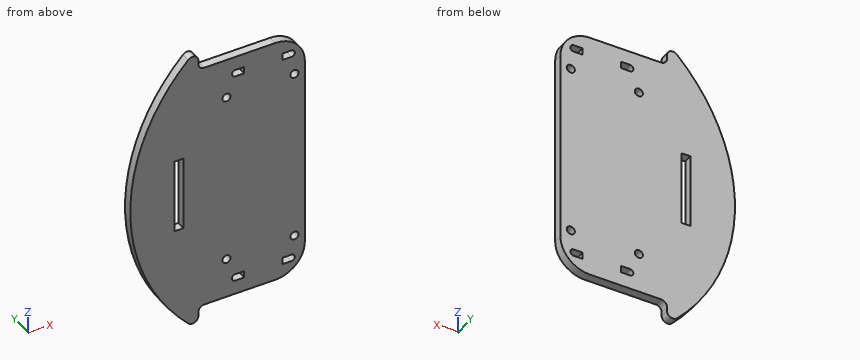
Autodesk Inventor part; units mm, degrees
ref_plane "YZ Plane" through (0, 0, 0) normal (1, 0, 0) x (0, 1, 0)
ref_plane "XZ Plane" through (0, 0, 0) normal (0, 1, 0) x (-1, 0, 0)
ref_plane "XY Plane" through (0, 0, 0) normal (0, 0, 1) x (1, 0, 0)
sketch "Boceto1" plane through (0, 0, 0) normal (0, 1, 0) x (-1, 0, 0)
  line L0 (3, 0) -> (33, 0)
  line L1 (36, -3) -> (36, -62)
  line L2 (33, -65) -> (3, -65)
  line L3 (0, -62) -> (0, -3)
  circle A0 centre (3.5, -61.5) radius 1.375
  arc A1 (36, -3) -> (33, 0) centre (33, -3) ccw
  arc A2 (3, 0) -> (0, -3) centre (3, -3) ccw
  arc A3 (0, -62) -> (3, -65) centre (3, -62) ccw
  arc A4 (33, -65) -> (36, -62) centre (33, -62) ccw
  circle A5 centre (26.5, -61.5) radius 1.375
  circle A6 centre (3.5, -3.5) radius 1.375
  circle A7 centre (26.5, -3.5) radius 1.375
  line L4 (36, 0) -> (0, 0)
  line L5 (0, 0) -> (0, 10)
  line L6 (0, 10) -> (36, 10)
  line L7 (36, 10) -> (36, 0)
  line L8 (36, -65) -> (0, -65)
  line L9 (0, -65) -> (0, -75)
  line L10 (0, -75) -> (36, -75)
  line L11 (36, -75) -> (36, -65)
  line L12 (7.5, 0) -> (20.5, 0)
  line L13 (20.5, 0) -> (20.5, 10)
  line L14 (20.5, 10) -> (7.5, 10)
  line L15 (7.5, 10) -> (7.5, 0)
  line L16 (7.5, 0) -> (20.5, 10) construction
  line L17 (20.5, 0) -> (7.5, 10) construction
  line L18 (7.5, -75) -> (20.5, -75)
  line L19 (20.5, -75) -> (20.5, -65)
  line L20 (20.5, -65) -> (7.5, -65)
  line L21 (7.5, -65) -> (7.5, -75)
  line L22 (7.5, -75) -> (20.5, -65) construction
  line L23 (20.5, -75) -> (7.5, -65) construction
  line L24 (36, -32.5) -> (0, -32.5)
  line L25 (36, 0) -> (36, -3)
  line L26 (0, 0) -> (0, -3)
  line L27 (0, -62) -> (0, -65)
  line L28 (36, -62) -> (36, -65)
  line L29 (36, -22.5) -> (49, -22.5)
  line L30 (49, -22.5) -> (49, -42.5)
  line L31 (49, -42.5) -> (36, -42.5)
  line L32 (36, -42.5) -> (36, -22.5)
  arc A8 (49, -42.5) -> (49, -22.5) centre (49, -32.5) ccw
  line L33 (20.5, 5.3) -> (23.5, 5.3)
  line L34 (23.5, 5.3) -> (23.5, 3)
  line L35 (23.5, 3) -> (20.5, 3)
  line L36 (20.5, 3) -> (20.5, 5.3)
  arc A9 (23.5, 3) -> (23.5, 5.3) centre (23.5, 4.15) ccw
  line L37 (14, 0) -> (14, -65)
  line L38 (7.5, 5.3) -> (4.5, 5.3)
  line L39 (4.5, 5.3) -> (4.5, 3)
  line L40 (4.5, 3) -> (7.5, 3)
  line L41 (7.5, 3) -> (7.5, 5.3)
  arc A10 (4.5, 5.3) -> (4.5, 3) centre (4.5, 4.15) ccw
  line L42 (20.5, -70.3) -> (23.5, -70.3)
  line L43 (23.5, -70.3) -> (23.5, -68)
  line L44 (23.5, -68) -> (20.5, -68)
  line L45 (20.5, -68) -> (20.5, -70.3)
  arc A11 (23.5, -70.3) -> (23.5, -68) centre (23.5, -69.15) ccw
  line L46 (4.5, -68) -> (7.5, -68)
  arc A12 (4.5, -68) -> (4.5, -70.3) centre (4.5, -69.15) ccw
  line L47 (7.5, -70.3) -> (4.5, -70.3)
  line L48 (4.5, -70.3) -> (4.5, -68)
  line L49 (7.5, -68) -> (7.5, -70.3)
  line L50 (36, 0) -> (49, 0)
  line L51 (49, 0) -> (49, -65)
  line L52 (49, -65) -> (36, -65)
  line L53 (36, -65) -> (36, 0)
  line L54 (44, -20) -> (41, -20)
  line L55 (41, -20) -> (41, -45)
  line L56 (41, -45) -> (44, -45)
  line L57 (44, -45) -> (44, -20)
  line L58 (36, 10) -> (36, 18)
  line L59 (36, -75) -> (36, -83)
  arc A13 (36, -83) -> (36, 18) centre (-7.9402, -32.5) ccw
  line L60 (0, -75) -> (-7, -75)
  line L61 (-7, -75) -> (-7, 10)
  line L62 (-7, 10) -> (0, 10)
  line L63 (0, 10) -> (0, -75)
  point P0 (14, 5)
  point P1 (14, -70)
  point P2 (36, -42.5)
  point P3 (7.5, -70.3)
  point P4 (20.5, -70.3)
  point P5 (7.5, 5.3)
  point P6 (20.5, 3)
  point P7 (44, -32.5)
  point P8 (36, -65)
  point P9 (44, -42.5)
  point P10 (41, -42.5)
  point P11 (41, -22.5)
  point P12 (44, -22.5)
  point P13 (49, -22.5)
  point P14 (59, -32.5)
  dimension "d0" = 36
  dimension "d1" = 65
  dimension "d2" = 2.75
  dimension "d3" = 3
  dimension "d4" = 3
  dimension "d5" = 3
  dimension "d6" = 3
  dimension "d7" = 3.5
  dimension "d8" = 3.5
  dimension "d11" = 23
  dimension "d14" = 58
  dimension "d17" = 10
  dimension "d18" = 10
  dimension "d19" = 13
  dimension "d20" = 10
  dimension "d21" = 13
  dimension "d22" = 10
  dimension "d26" = 7.5
  dimension "d30" = 20
  dimension "d31" = 13
  dimension "d32" = 3
  dimension "d33" = 2.3
  dimension "d34" = 3
  dimension "d35" = 1.15
  dimension "d36" = 13
  dimension "d37" = 3
  dimension "d38" = 25
  dimension "d39" = 5
  dimension "d42" = 8
  dimension "d43" = 8
  dimension "d46" = 7
extrude "Extrusión1" add sketch "Boceto1" along normal blind 3 contours L4 L5 L6 L15 L38 A10 L40 L0 | L0 L37 L24 L3 A2 | A2 L26 L4 | L15 L6 L13 L0 | L0 A1 L1 L24 L37 | L24 L37 L2 A3 L3 | L13 L35 A9 L33 L6 L7 L4 L0 | L24 L1 A4 L2 L37 | A3 L8 L27 | L4 L25 A1 | L1 L29 L55 L31 | L2 L19 L10 L21 | L2 L21 L46 A12 L47 L10 L9 L8 | L25 L50 L51 L29 L57 L54 L55 L1 | L7 L58 A13 A8 L51 L50 | L31 L55 L56 L57 L51 L52 L28 L1 | L2 L8 L11 L10 L19 L42 A11 L44 | L29 L57 L31 L55 | L28 L8 A4 | L30 L31 L57 L29 | A8 L30 | L52 L51 A8 A13 L59 L11
fillet "Empalme1" radius 10 2 edges at (0, 1.5, -75) (0, 1.5, 10)
extrude "Extrusión2" cut sketch "Boceto1" along normal blind 3 contours L29 L57 L31 L55
fillet "Empalme2" radius 2 4 edges at (-36, 1.5, -83) (-36, 1.5, 18) (-36, 1.5, 10) (-36, 1.5, -75)
equation "\"d18\" = d17"
equation "\"d21\" = d19"
equation "\"d22\" = d20"
equation "\"d36\" = d31"
properties part number "Parte inferior"
Input: part model. Units: mm. Frame: model coordinates. Coordinates: 2 decimals unless noted, no trailing zeros. Loops run counter-clockwise (first coordinate to the right, second up) from the corner with the lowest first, then second, coordinate; pieces in that order, holes last. Notation, with made-up numbers: (23, 34) -> (41, 34) arc R16 ccw to (41, 48) -> close; hole circle Ø2 at (35.5, 46). An arc over 180 degrees is marked (long way). Write each question's results on one line, items separated by ' | '. Start each with the question number.
Q1. Section B-B, the plane x = -26.5. Return the cut outline in (y, z) (3 decimals), plus the area to 4 significant figures.
Q2. Section C-C, the plane z = 4.15. Return the cut outline in (x, y), plus the area to 3 significant figures.
Q3. Section A-A, the plane z = -23. Return the cut outline in (x, y), plus the area to 3 significant figures.
Q4. Pin query (flat end, axial travel): pin 1 (3.5 mm diameter, centred on x = -26.5, z = -61.5, fed in from +Y); pin 2 (1.5 mm diameter, centred on x = -22.5, y = 1, fed in from +Z); pin 3 (1.5 mm diameter, centred on x = -6, y = 1.5, fed in from +Z); pin 4 (1.2 mm diameter, centred on y = 1, z = 4, fed in from -X). Return the tip coordinate at first contact, or that it passes through.
Q5. Section D-D, the plane y = 0.7. State how many separate pieces and enclosed holes the cut face has, plus the area to 3 significant figures.
Q6. Ray query, line 1 (Z direction, x = -26.5, y = 1.15) (3 decimals); line 2 (Z direction, x = -3.5, y = 1.85) (3 decimals); line 3 (Z direction, x = -24, y = 2.8). Return the intervals inside material, ascending. Write a range as from..to.
Found:
1) outline: (0, -75) -> (3, -75) -> (3, -62.875) -> (0, -62.875) -> close; (0, -60.125) -> (3, -60.125) -> (3, -4.875) -> (0, -4.875) -> close; (0, -2.125) -> (3, -2.125) -> (3, 10) -> (0, 10) -> close | area: 238.5 mm2
2) outline: (-48.08, 0) -> (-24.65, 0) -> (-24.65, 3) -> (-48.08, 3) -> close; (-20.5, 0) -> (-7.5, 0) -> (-7.5, 3) -> (-20.5, 3) -> close; (-3.35, 0) -> (-0.9, 0) -> (-0.9, 3) -> (-3.35, 3) -> close | area: 117 mm2
3) outline: (-58.32, 0) -> (-44, 0) -> (-44, 3) -> (-58.32, 3) -> close; (-41, 0) -> (0, 0) -> (0, 3) -> (-41, 3) -> close | area: 166 mm2
4) pin 1: y = 3 | pin 2: z = 10 | pin 3: z = 9.46 | pin 4: x = -48.56
5) separate pieces: 1 | enclosed holes: 9 | area: 4,490 mm2
6) line 1: -75..-62.875, -60.125..-4.875, -2.125..10 | line 2: -72.599..-69.718, -68.582..-62.875, -60.125..-4.875, -2.125..3.582, 4.718..7.599 | line 3: -75..-70.19, -68.11..3.11, 5.19..10
